Input: part model. Units: mm. Frame: model coordinates. Coordinates: 2 decimals unless noted, no trailing zeros. Order: outer loops, then holes, each group sorted by start corner. A loop starts at its lowest first (then second) coordinate and runs counter-clockwise, first axis right, second up. Notation, with made-up numbers: (31, -37) -> (57, -37) arc R28 ccw to (57, -10) -> close; hole circle Ø7 at (-5.5, -25). An arc over 180 degrees is marked (long way). Write each question's results on one line, items separated by ' | '.
```python
from build123d import *

# Parameters (mm, degrees)
F0_W     = 38.1
F0_H     = 38.1
F1_DEPTH = 0.79375
F2_W     = 38.1
F2_H     = 38.1
F2_W_2   = 34.925
F2_H_2   = 34.925
F3_DEPTH = 6.35
F4_W     = 1.1048951419
F4_H     = 2.9129034374
F4_W_2   = 5.5244707037
F4_H_2   = 2.109343739
F4_W_3   = 2.1220554633
F4_H_3   = 7.4329261261
F4_W_4   = 3.8873708525
F4_H_4   = 4.1415788532
F4_W_5   = 2.5213125627
F4_H_5   = 3.0267448165
F5_DEPTH = 4.445
F6_R     = 1.3326175267
F6_R_2   = 1.27
F7_DEPTH = 0.396875


with BuildPart() as f1:
    # F0 (on Top) → F1 (new body)
    with BuildSketch(Plane.XY):
        with Locations((-0.3095176071, -5.7596102857)):
            Rectangle(F0_W, F0_H)
    extrude(amount=F1_DEPTH)

    # F2 (on face) → F3 (join)
    with BuildSketch(Plane.XY.offset(0.79375)):
        with Locations((-0.3095176071, -5.7596102857)):
            Rectangle(F2_W, F2_H)
        with Locations((-0.3095176071, -5.7596102857)):
            Rectangle(F2_W_2, F2_H_2, mode=Mode.SUBTRACT)
    extrude(amount=F3_DEPTH)

    # F4 (on face) → F5 (join)
    with BuildSketch(Plane.XY.offset(0.79375)):
        Polygon((-12.6920176071, 6.6228897143), (-12.6920176071, -23.2221102857), (-10.1520176071, -23.2221102857), (-10.1520176071, -19.9179127812), (-10.1520176071, -12.9872104153), (-10.1520176071, 0.3719671222), (-10.1520176071, 5.3942142986), (-10.1520176071, 6.6228897143), align=None)
        Polygon((0.5091035802, 6.6228897143), (-10.1520176071, 6.6228897143), (-10.1520176071, 5.3942142986), (-0.5957915617, 5.3942142986), (0.5091035802, 5.3942142986), align=None)
        Polygon((-10.1520176071, -12.9872104153), (-10.1520176071, -19.9179127812), (-0.3095176071, -19.9179127812), (4.7704823929, -19.9179127812), (4.7704823929, -12.9872104153), (-0.5957915617, -12.9872104153), align=None)
        Polygon((-0.5957915617, 5.3942142986), (-10.1520176071, 5.3942142986), (-10.1520176071, 0.3719671222), (-10.1520176071, -12.9872104153), (-0.5957915617, -12.9872104153), (-0.5957915617, 0.3719671222), (-0.5957915617, 2.4813108612), align=None)
        Polygon((4.7704823929, -19.9179127812), (-0.3095176071, -19.9179127812), (-0.3095176071, -23.2221102857), (9.8504823929, -23.2221102857), (9.8504823929, -19.9179127812), align=None)
        with Locations((-0.0433439907, 3.9377625799)):
            Rectangle(F4_W, F4_H)
        Polygon((0.5091035802, 2.4813108612), (-0.5957915617, 2.4813108612), (-0.5957915617, 0.3719671222), (4.3260116892, 0.3719671222), (4.3260116892, 2.4813108612), (0.9108832403, 2.4813108612), align=None)
        with Locations((7.0882470411, 1.4266389917)):
            Rectangle(F4_W_2, F4_H_2)
        Polygon((9.8504823929, 2.4813108612), (9.8504823929, 0.3719671222), (9.9509269296, 0.3719671222), (12.0729823929, 0.3719671222), (12.0729823929, 2.4813108612), align=None)
        with Locations((11.0119546612, -3.3444959408)):
            Rectangle(F4_W_3, F4_H_3)
        Polygon((17.1529823929, -14.3934395164), (17.1529823929, -12.9872104153), (12.3616074508, -12.9872104153), (9.8504823929, -12.9872104153), (9.8504823929, -14.3934395164), align=None)
        with Locations((15.2092969666, 9.6321002878)):
            Rectangle(F4_W_4, F4_H_4)
        with Locations((4.3130695121, -4.8578686547)):
            Rectangle(F4_W_5, F4_H_5)
    extrude(amount=F5_DEPTH)

    # F6 (on face) → F7 (cut)
    with BuildSketch(Plane.XY.offset(0.79375)):
        with Locations((13.801550063, -19.3494927589)):
            Circle(F6_R)
        with Locations((-15.1696396893, -20.454704795)):
            Circle(F6_R_2)
    extrude(amount=-F7_DEPTH, mode=Mode.SUBTRACT)


solid = f1.part
```
(1) Cut plane A-A, the plane z = 6. Return loops of the section in (x, y), plus the area to 3 significant figures.
Return value:
outline: (-19.36, -24.81) -> (18.74, -24.81) -> (18.74, 13.29) -> (-19.36, 13.29) -> close; hole (-17.77, -23.22) -> (17.15, -23.22) -> (17.15, 11.7) -> (-17.77, 11.7) -> close | area: 232 mm2
(2) Pin query (flat end, axial travel): P1, Ø8, axis at x = -0.5, y = -9.5, coming from the +Z side; P2, Ø1, axis at x = -6.5, y = -21, coming from the +Z side. Return the tip coordinate at first contact, or that it passes through.
Return value:
P1: z = 5.24 | P2: z = 0.79
(3) Mould query, pull axis X, two halves, no side actions, for faces 1 (the face through (-1, 13.29, 4)), 2 (the face through (18.74, -6, 4)), 3 (the face through (9.85, -22, 3)), 4 (the face through (-19.36, -6, 4)). Classes: +X half, -X half, draft (parallel to the pull), parting line (faces both ways), or undercut.
Return value:
face 1: draft | face 2: +X half | face 3: undercut | face 4: -X half
(4) Line query: line 1 along Y through (x, z) = (2, 3.25); line 2 along X through (y, z) = (-5.5, 3.75); line 3 along Y through (x, z) = (-5, 1.5). Output: solid intervals per line, ascending. Write a range as from..to.
Return value:
line 1: -24.81..-12.99, 0.37..2.48, 11.7..13.29 | line 2: -19.36..-17.77, -12.69..-0.6, 3.05..5.57, 9.95..12.07, 17.15..18.74 | line 3: -24.81..-23.22, -19.92..6.62, 11.7..13.29
(5) Cut plane D-D, the plane z = 1.75. Count the separate pieces of the cut face and the enclosed holes in it, plus the area to 3 significant figures.
Return value:
separate pieces: 2 | enclosed holes: 2 | area: 713 mm2
(6) Cut plane C-C, the plane x = 11. Return loops of the section in (y, z), plus the area to 3 significant figures.
Return value:
outline: (-24.81, 0) -> (13.29, 0) -> (13.29, 7.14) -> (11.7, 7.14) -> (11.7, 0.79) -> (2.48, 0.79) -> (2.48, 5.24) -> (-7.06, 5.24) -> (-7.06, 0.79) -> (-12.99, 0.79) -> (-12.99, 5.24) -> (-14.39, 5.24) -> (-14.39, 0.79) -> (-23.22, 0.79) -> (-23.22, 7.14) -> (-24.81, 7.14) -> close | area: 99.1 mm2
(7) Cut plane B-B, the plane y = -11.5. Return loops of the section in (x, z).
Return value:
outline: (-19.36, 0) -> (18.74, 0) -> (18.74, 7.14) -> (17.15, 7.14) -> (17.15, 0.79) -> (-0.6, 0.79) -> (-0.6, 5.24) -> (-12.69, 5.24) -> (-12.69, 0.79) -> (-17.77, 0.79) -> (-17.77, 7.14) -> (-19.36, 7.14) -> close
